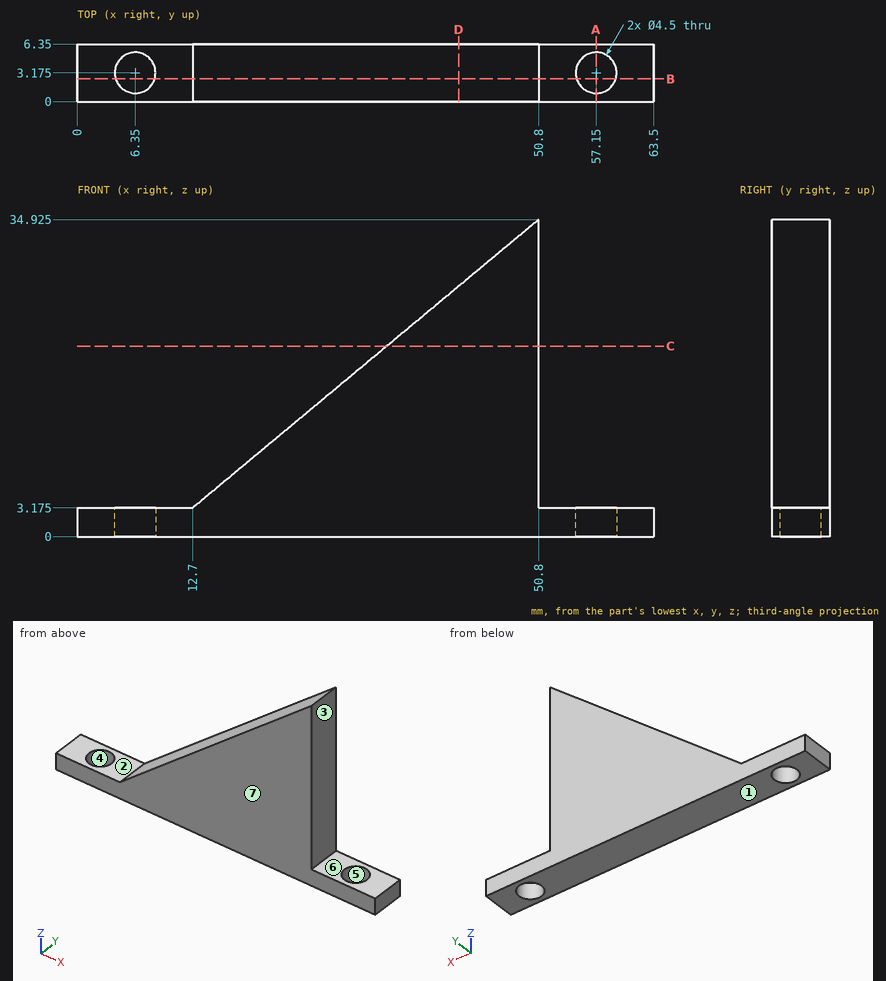
Part print with two shaded views. Sizes in mm from the minimum x, y, z corner. A direction names the side the tool comes from. Round coordinates to 2 decimals unless told otherwise and drop trailing zeros. Order: outer loops, then holes, each group sorted by start corner. A loop starts at its lowest first (then second) coordinate and runs counter-clockwise, first axis right, second up. Notation, with made-up numbers: M 63,35.5 L 105,35.5 A29 ccw 105,72.5 Z; hole C 57.5,68.25 d8. An arc over 180 degrees is marked long. Put each result on its own line as item: value. Start each with the question number.
1. Drop flat-ended pins along their axis: pin 1 (1.9 mm diameter, centred on x = 54, y = 3.5, fed in from +Z) (3 decimals); pin 2 (1 mm diameter, centred on x = 37.5, y = 2.5, fed in from +Z); pin 3 (3 mm diameter, centred on y = 1.5, z = 11.5, fed in from +X). Give the stop position or say it passes through.
2. Slice it at C-C on z = 21. List the corners of the cut face in (x, y), then the cut area to 3 significant figures.
3. Drill centre lines: probe 1 along Y at (x, z) = (57.15, 1.8) (3 decimals); probe 2 along Z at (x, y) = (11, 4) (3 decimals); probe 3 along X at (y, z) = (4.25, 29). Where is each one in solid material? Low to high. Write a range as [from, to].
4. Two-plate mould, pull along Y, no slides. Class the marked faces 4, 5, 6 and 7: +Y half, -Y half, draft (parallel to the pull), parting line (faces both ways), or undercut.
5. Slice it at A-A on x = 57.15. List the corners of the cut face in (y, z) (3 decimals), then the cut area to 3 significant figures.
6. Slice it at B-B on y = 2.5. List the corners of the cut face in (x, z) (3 decimals), then the cut area to 3 significant figures.
7. Slice it at D-D on x = 42. List the corners of the cut face in (y, z).
8. Tool access for the marked faces 1, 2 and 3: list every direction of +Z, -Z, +X, -X, +Y, -Y with a clear straight run to the whole face (end or side of a thin tool).
Findings:
1. pin 1: z = 3.175
1. pin 2: z = 24.26
1. pin 3: x = 50.8
2. outline: M 34.09,0 L 50.8,0 L 50.8,6.35 L 34.09,6.35 Z
2. area: 106 mm2
3. probe 1: [0, 0.925], [5.425, 6.35]
3. probe 2: [0, 3.175]
3. probe 3: [43.69, 50.8]
4. face 4: undercut
4. face 5: undercut
4. face 6: draft
4. face 7: -Y half
5. outline: M 0,0 L 0.925,0 L 0.925,3.175 L 0,3.175 Z; M 5.425,0 L 6.35,0 L 6.35,3.175 L 5.425,3.175 Z
5. area: 5.87 mm2
6. outline: M 0,0 L 4.204,0 L 4.204,3.175 L 0,3.175 Z; M 8.496,0 L 55.004,0 L 55.004,3.175 L 50.8,3.175 L 50.8,34.925 L 12.7,3.175 L 8.496,3.175 Z; M 59.296,0 L 63.5,0 L 63.5,3.175 L 59.296,3.175 Z
6. area: 779 mm2
7. outline: M 0,0 L 6.35,0 L 6.35,27.59 L 0,27.59 Z
8. face 1: -Z, +X, -X, +Y, -Y
8. face 2: +Z, -X, +Y, -Y
8. face 3: +Z, +X, +Y, -Y
